Verification items for the finished model (mm, model axes). A direction names the side the tool comes from. Round coordinates to 2 decimals unless told otherwise and drop trailing zeros. Loops run counter-clockwise (first coordinate to the right, second up) from the corner with the lowest first, then second, coordinate; pieces in that order, holes last. Notation, with made-up numbers: M 81,23.25 L 93,23.25 A22 ccw 93,35.25 Z; hole C 57.5,65.25 d8. An arc over 180 degrees is marked long. One line per item, written item: value.
from build123d import *

# Parameters (mm, degrees)
F0_W      = 100
F0_H      = 100
F1_DEPTH  = 200
F2_W      = 92
F2_H      = 92
F3_DEPTH  = 200
F4_R      = 5
F5_DEPTH  = 4
F7_DEPTH  = 4
F4_R_2    = 7
F8_DEPTH  = 20
F11_DEPTH = 1
F12_DEPTH = 20
F13_W     = 216.226272
F13_H     = 124.404148
F14_DEPTH = 304.8


with BuildPart() as f1:
    # F0 (on Front) → F1 (new body)
    with BuildSketch(Plane.XZ):
        with Locations((50, 50)):
            Rectangle(F0_W, F0_H)
    extrude(amount=-F1_DEPTH)

    # F2 (on face) → F3 (cut)
    with BuildSketch(Plane.XZ):
        with Locations((50, 50)):
            Rectangle(F2_W, F2_H)
    extrude(amount=-F3_DEPTH, mode=Mode.SUBTRACT)

    # F4 (on face) → F5 (cut)
    with BuildSketch(Plane.YZ.offset(100)):
        with Locations((50, 50)):
            Circle(F4_R)
        with Locations((100, 50)):
            Circle(F4_R)
        with Locations((150, 50)):
            Circle(F4_R)
    extrude(amount=-F5_DEPTH, mode=Mode.SUBTRACT)

    # F6 (on face) → F7 (cut)
    with BuildSketch(Plane(origin=(0, 0, 0), x_dir=(0, -1, 0), z_dir=(-1, 0, 0))):
        Polygon((-50, 50.4), (-50.85, 50.4), (-50.85, 49.6), (-49.15, 49.6), (-49.15, 50.4), align=None)
        Polygon((-100, 50.4), (-100.85, 50.4), (-100.85, 49.6), (-99.15, 49.6), (-99.15, 50.4), align=None)
        Polygon((-150, 50), (-150, 49.6), (-149.15, 49.6), (-149.15, 50.4), (-150, 50.4), align=None)
        Polygon((-150.85, 49.6), (-150, 49.6), (-150, 50), (-150, 50.4), (-150.85, 50.4), align=None)
    extrude(amount=-F7_DEPTH, mode=Mode.SUBTRACT)

    # F4 (on face) → F8 (join)
    with BuildSketch(Plane.YZ.offset(100)):
        with Locations((50, 50)):
            Circle(F4_R_2)
        with Locations((50, 50)):
            Circle(F4_R, mode=Mode.SUBTRACT)
        with Locations((100, 50)):
            Circle(F4_R_2)
        with Locations((100, 50)):
            Circle(F4_R, mode=Mode.SUBTRACT)
        with Locations((150, 50)):
            Circle(F4_R_2)
        with Locations((150, 50)):
            Circle(F4_R, mode=Mode.SUBTRACT)
    extrude(amount=F8_DEPTH)

    # F10 (on face) → F11 (join)
    with BuildSketch(Plane(origin=(96, 0, 0), x_dir=(0, -1, 0), z_dir=(-1, 0, 0))):
        with BuildLine():
            Line((-45.069934, 49.166667), (-49.99933, 49.166667))
            Line((-49.99933, 49.166667), (-54.930066, 49.166667))
            ThreePointArc((-54.930066, 49.166667), (-50, 45), (-45.069934, 49.166667))
        make_face()
        with BuildLine():
            Line((-95.069934, 49.166667), (-99.99933, 49.166667))
            Line((-99.99933, 49.166667), (-104.930066, 49.166667))
            ThreePointArc((-104.930066, 49.166667), (-100, 45), (-95.069934, 49.166667))
        make_face()
        with BuildLine():
            Line((-145.069934, 49.166667), (-149.99933, 49.166667))
            Line((-149.99933, 49.166667), (-154.930066, 49.166667))
            ThreePointArc((-154.930066, 49.166667), (-150, 45), (-145.069934, 49.166667))
        make_face()
    extrude(amount=-F11_DEPTH)

    # F9 (on face) → F12 (join)
    with BuildSketch(Plane.YZ.offset(120)):
        with BuildLine():
            Line((47.001097, 54.000823), (47.001097, 56.325076))
            ThreePointArc((47.001097, 56.325076), (46.257829, 44.084245), (57, 50))
            ThreePointArc((57, 50), (55.91608, 53.741657), (53, 56.324555))
            Line((53, 56.324555), (53, 54))
            ThreePointArc((53, 54), (54.472136, 52.236068), (55, 50))
            ThreePointArc((55, 50), (47.763319, 45.528171), (47.001097, 54.000823))
        make_face()
        with BuildLine():
            Line((103, 56.324555), (103, 54))
            ThreePointArc((103, 54), (99.999314, 45), (97.001097, 54.000823))
            Line((97.001097, 54.000823), (97.001097, 56.325076))
            ThreePointArc((97.001097, 56.325076), (99.999393, 43), (103, 56.324555))
        make_face()
        with BuildLine():
            Line((153, 56.324555), (153, 54))
            ThreePointArc((153, 54), (149.999314, 45), (147.001097, 54.000823))
            Line((147.001097, 54.000823), (147.001097, 56.325076))
            ThreePointArc((147.001097, 56.325076), (149.999393, 43), (153, 56.324555))
        make_face()
    extrude(amount=F12_DEPTH)

    # F13 (on face) → F14 (cut)
    with BuildSketch(Plane(origin=(96, 0, 0), x_dir=(0, -1, 0), z_dir=(-1, 0, 0))):
        with Locations((-99.291925, 46.610653)):
            Rectangle(F13_W, F13_H)
    extrude(amount=-F14_DEPTH, mode=Mode.SUBTRACT)


solid = f1.part
(1) Thickness scan on L1, parallel to Z at x = 42.5, y = 79; L2, parallel to X at y = 183, z = 74.5. Record the ranges inside material, lowest first. Write a range as from..to.
Completed:
L1: z = 0..4, 96..100
L2: x = 0..4
(2) Sectioned sample at A-A on x = 40. Enter the section's corners in (y, z), and give its area (3 significant figures).
Completed:
outline: M 0,0 L 200,0 L 200,4 L 0,4 Z; M 0,96 L 200,96 L 200,100 L 0,100 Z
area: 1,600 mm^2
(3) Tool access check on faces 1 (the face through (96, 101, 2)), 2 (the face through (4, 99, 49)). Record the directions out of +Z, -Z, +X, -X, +Y, -Y that give a thin tool (end or side, any length) a straight path to the whole face; none if there is none.
Completed:
face 1: +Z, -Z, +X, +Y, -Y
face 2: +X, +Y, -Y
(4) Sectioned sample at C-C on z = 41.5. Enter the section's corners in (x, y), and give its area (3 significant figures).
Completed:
outline: M 0,0 L 4,0 L 4,200 L 0,200 Z
area: 800 mm^2
(5) Mould release check, pull along Z, two halves, no side actions. Record for faces 3 (the face through (49, 99, 96)), 4 (the face through (0, 99, 49)), 5 (the face through (47, 99, 100)): +Z half, -Z half, draft (parallel to the pull), parting line (faces both ways), or undercut.
Completed:
face 3: undercut
face 4: draft
face 5: +Z half
(6) Sectioned sample at B-B on y = 118. Enter the section's corners in (x, z), and give its area (3 significant figures).
Completed:
outline: M 0,0 L 96,0 L 96,4 L 4,4 L 4,96 L 96,96 L 96,100 L 0,100 Z
area: 1,140 mm^2
